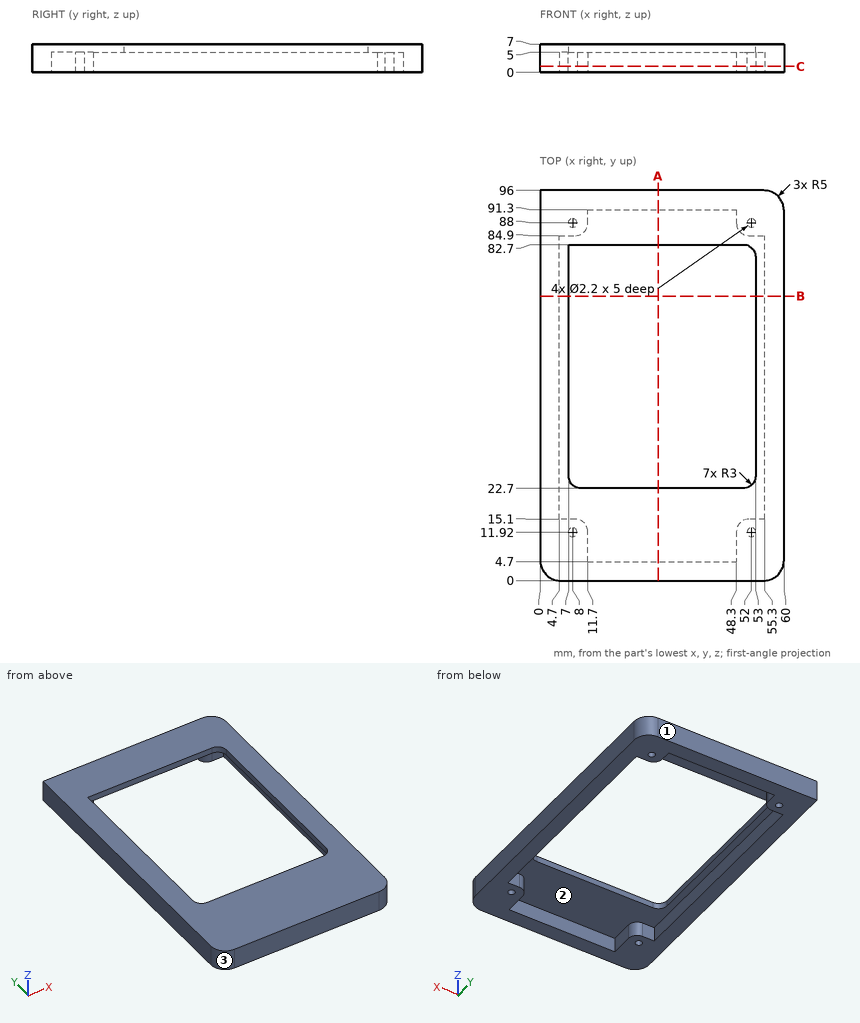
Design review of the part shown in the three views and the two pictorial views. Dimensions are in mm from the part's minimum x, y and z. Coordinates: 2 decimals unless noted, no trailing zeros. Write each loop counter-clockwise with the first axis right and the second up, starting at its lowest first coordinate (ties: lowest second). Pieces come first, ordered by that corner, then holes. Notation, with made-up numbers: (54.5, -35) - (101.5, -35) arc R10 cw to (101.5, -31) - close; hole circle Ø8 at (8, -7.75). An arc over 180 degrees is marked (long way). Write item = value, one per line.
(1) Consider section C-C, the plane z = 1.5. Give the boundary of the cut face in (x, y).
Result sheet:
outline = (0, 5) arc R5 ccw to (5, 0) - (55, 0) arc R5 ccw to (60, 5) - (60, 91) arc R5 ccw to (55, 96) - (0, 96) - close; hole (4.7, 15.1) - (8.7, 15.1) arc R3 cw to (11.7, 12.1) - (11.7, 4.7) - (48.3, 4.7) - (48.3, 12.1) arc R3 cw to (51.3, 15.1) - (55.3, 15.1) - (55.3, 84.9) - (51.3, 84.9) arc R3 cw to (48.3, 87.9) - (48.3, 91.3) - (11.7, 91.3) - (11.7, 87.9) arc R3 cw to (8.7, 84.9) - (4.7, 84.9) - close; hole circle Ø2.2 at (8, 11.92); hole circle Ø2.2 at (8, 88); hole circle Ø2.2 at (52, 11.92); hole circle Ø2.2 at (52, 88)
(2) For P1, Ø1.1, axis at x = 52.5, y = 88, coming from the -Z side, flat-tipped, find the tip position at first contact; note if it passes through.
Result sheet:
P1 = 5
(3) Consider section A-A, the plane x = 29. Give the boundary of the cut face in (y, z).
Result sheet:
outline = (0, 0) - (4.7, 0) - (4.7, 5) - (22.7, 5) - (22.7, 7) - (0, 7) - close; (82.7, 5) - (91.3, 5) - (91.3, 0) - (96, 0) - (96, 7) - (82.7, 7) - close
(4) Mouldability with a two-part tool opening along X and no side actions: class the marked faces 1, 2 and 3 as pulls with the +X half, pulls with the -X half, needs draft (parallel to the pull), parting line crosses it, or undercut.
Result sheet:
face_1 = needs draft
face_2 = undercut
face_3 = pulls with the -X half
(5) For line 1 (Y direction, x = 52, z = 2.3); line 2 (X direction, y = 31, z = 1.5); line 3 (Y direction, x = 15, z = 0.75), list the stretches that pass through material, from the lowest coordinate up. Write a range as [from, to].
Result sheet:
line_1 = [0, 10.82], [13.02, 15.1], [84.9, 86.9], [89.1, 96]
line_2 = [0, 4.7], [55.3, 60]
line_3 = [0, 4.7], [91.3, 96]
(6) Consider section B-B, the plane y = 70. Give the boundary of the cut face in (x, z), then the cut area to 3 significant figures.
Result sheet:
outline = (0, 0) - (4.7, 0) - (4.7, 5) - (7, 5) - (7, 7) - (0, 7) - close; (53, 5) - (55.3, 5) - (55.3, 0) - (60, 0) - (60, 7) - (53, 7) - close
area = 75.0 mm^2
